Geometry: see drawing. Coordinates: mm, zero at the bounding-box minimum. Give positions to 0.01 mm unless a question says otherwise; leave off trailing zeros. Write each loop counter-clockwise with the first axis right and the second up, starting at its lowest first coordinate (ties: lowest second). Pieces come first, ordered by that corner, then holes. Notation, with made-up numbers: M 18,29 L 46,29 A30 cw 46,55 Z; hole C 3,78.5 d8. An arc over 180 degrees is marked long. Use one line per item in the form item = value. Start each with the question number.
Item 1: Contact query for a flat-ended pin moving along its axis: P1, Ø9.5, axis at x = 189.5, y = 11, coming from the -Z side. Output: stop coordinate, or through.
Item 2: Section query A-A on z = 51. Return loops of the section in (x, y), then the cut area to 4 significant figures.
Item 3: Section query B-B on y = 13.25. Return loops of the section in (x, z).
Item 4: Section query C-C on x = 201. Return loops of the section in (y, z).
Item 5: Material intervals for line 1 along Z through (x, y) = (49, 13.25); line 2 along X through (y, z) = (8.5, 114.5), sorted ascending. Write a range as from..to.
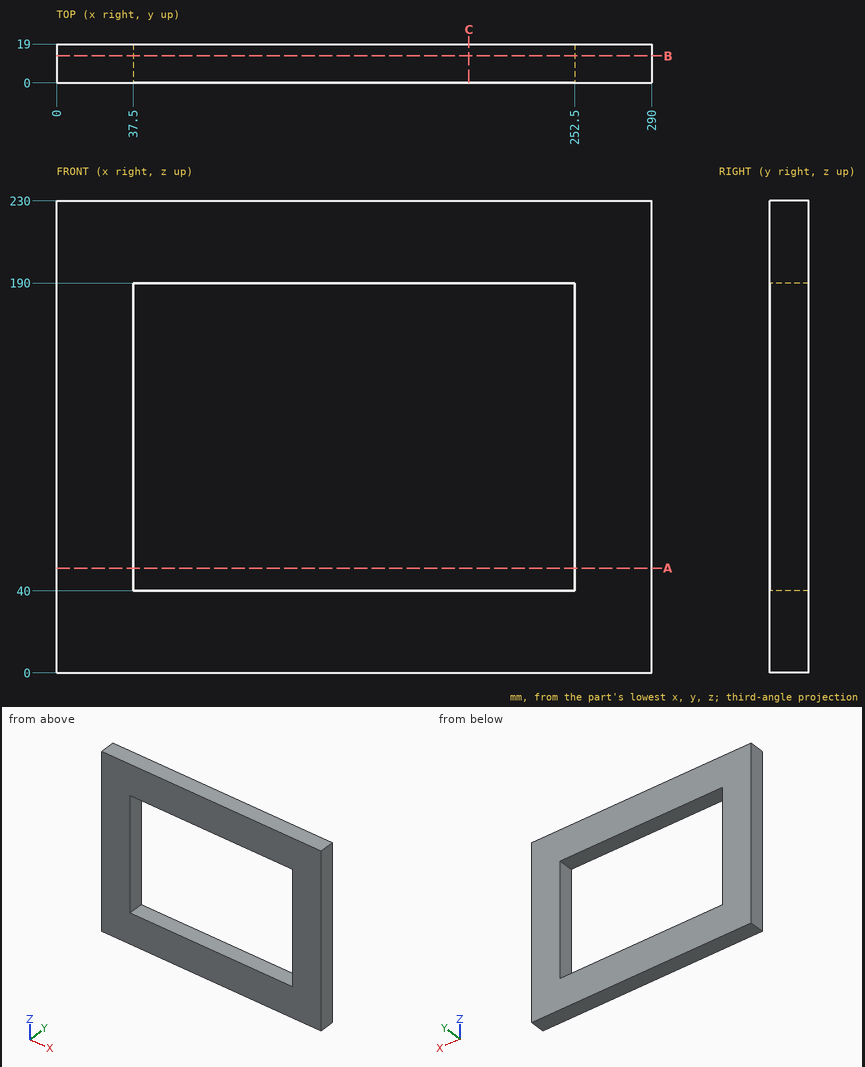
Answer sheet:
q1.P1 = 0
q2.outline = M 0,0 L 37.5,0 L 37.5,19 L 0,19 Z; M 252.5,0 L 290,0 L 290,19 L 252.5,19 Z
q2.area = 1,425 mm2
q3.outline = M 0,0 L 290,0 L 290,230 L 0,230 Z; hole M 37.5,40 L 252.5,40 L 252.5,190 L 37.5,190 Z
q4.outline = M 0,0 L 19,0 L 19,40 L 0,40 Z; M 0,190 L 19,190 L 19,230 L 0,230 Z
q5.line_1 = 0..40, 190..230
q5.line_2 = 0..37.5, 252.5..290
